Part model, mm, in its own coordinate system. Face numbers are marked on the shaded views. Give positions to 0.01 mm unless a question says otherwise; leave off trailing zeros. Write each loop counter-clockwise with the first axis right and the second up, starting at its lowest first coordinate (ties: lowest second). Pieces come first, ordered by that corner, then holes. Notation, with made-up numbers: M 88.25,-32.5 L 128.25,-32.5 A18 ccw 128.25,-26.5 Z; hole C 13,12 d1. An arc over 180 degrees is marked long. Use a Markdown table: item, result. Add a question column.
from build123d import *

# Parameters (mm, degrees)
F0_R         = 75.9313176518
F0_R_2       = 63.6217413668
F1_DEPTH     = 8.128
F2_DEPTH     = 11.43
F3_R         = 8.1097941577
F4_DEPTH     = 100.33
F5_DEPTH     = 117.094
F6_R         = 8.1153
F7_DEPTH     = 85.852
F8_DEPTH     = 117.094
F9_T2_ANGLE  = 87.3226513318
F9_T4_ANGLE  = 87.3226513318
F9_T6_ANGLE  = 87.3226513318
F9_T8_ANGLE  = 87.3226513318
F10_T2_ANGLE = 92.5127162525
F10_T4_ANGLE = 92.5127162525
F10_T6_ANGLE = 92.5127162525
F10_T8_ANGLE = 92.5127162525


# Not quite as in the source:
# - a fillet or chamfer that OpenCascade refuses, or shapes differently, is made with other operations: its cross-section is extruded or revolved along the edge and cut away or added


with BuildPart() as f1:
    # F0 (on Top) → F1 (new body)
    with BuildSketch(Plane.XY):
        Circle(F0_R)
        Circle(F0_R_2, mode=Mode.SUBTRACT)
        Circle(F0_R_2)
    extrude(amount=-F1_DEPTH)

    # F0 (on Top) → F2 (join)
    with BuildSketch(Plane.XY):
        Circle(F0_R)
        Circle(F0_R_2, mode=Mode.SUBTRACT)
    extrude(amount=F2_DEPTH)

    # F3 (on Right) → F4 (cut)
    with BuildSketch(Plane.YZ):
        with Locations((0, 11.5122310817)):
            Circle(F3_R)
    extrude(amount=-F4_DEPTH, mode=Mode.SUBTRACT)

    # F3 (on Right) → F5 (cut)
    with BuildSketch(Plane.YZ):
        with Locations((0, 11.5122310817)):
            Circle(F3_R)
    extrude(amount=F5_DEPTH, mode=Mode.SUBTRACT)

    # F6 (on Front) → F7 (cut)
    with BuildSketch(Plane.XZ):
        with Locations((0, 11.1844760826)):
            Circle(F6_R)
    extrude(amount=-F7_DEPTH, mode=Mode.SUBTRACT)

    # F6 (on Front) → F8 (cut, symmetric)
    with BuildSketch(Plane.XZ):
        with Locations((0, 11.1844760826)):
            Circle(F6_R)
    extrude(amount=F8_DEPTH, both=True, mode=Mode.SUBTRACT)

    # F9: fillet of radius 2.54 on 4 edges, made by hand

    # F9_s1 → F9_t2 (revolve, cut)
    with BuildSketch(Plane(origin=(0, 0, 0), x_dir=(0, 0, 1), z_dir=(-0.999726726, -0.0233767669, 0))):
        with BuildLine():
            ThreePointArc((8.89, -75.9313176518), (10.6860512242, -75.187368876), (11.43, -73.3913176518))
            Line((11.43, -73.3913176518), (11.43, -75.9313176518))
            Line((11.43, -75.9313176518), (8.89, -75.9313176518))
        make_face()
    revolve(axis=Axis((0, 0, 11.43), (0, 0, 1)), revolution_arc=F9_T2_ANGLE, mode=Mode.SUBTRACT)

    # F9_s3 → F9_t4 (revolve, cut)
    with BuildSketch(Plane(origin=(0, 0, 0), x_dir=(0, 0, 1), z_dir=(-0.0233475312, 0.9997274092, 0))):
        with BuildLine():
            ThreePointArc((8.89, -75.9313176518), (10.6860512242, -75.187368876), (11.43, -73.3913176518))
            Line((11.43, -73.3913176518), (11.43, -75.9313176518))
            Line((11.43, -75.9313176518), (8.89, -75.9313176518))
        make_face()
    revolve(axis=Axis((0, 0, 11.43), (0, 0, 1)), revolution_arc=F9_T4_ANGLE, mode=Mode.SUBTRACT)

    # F9_s5 → F9_t6 (revolve, cut)
    with BuildSketch(Plane(origin=(0, 0, 0), x_dir=(0, 0, 1), z_dir=(0.999726726, 0.0233767669, 0))):
        with BuildLine():
            ThreePointArc((8.89, -75.9313176518), (10.6860512242, -75.187368876), (11.43, -73.3913176518))
            Line((11.43, -73.3913176518), (11.43, -75.9313176518))
            Line((11.43, -75.9313176518), (8.89, -75.9313176518))
        make_face()
    revolve(axis=Axis((0, 0, 11.43), (0, 0, 1)), revolution_arc=F9_T6_ANGLE, mode=Mode.SUBTRACT)

    # F9_s7 → F9_t8 (revolve, cut)
    with BuildSketch(Plane(origin=(0, 0, 0), x_dir=(0, 0, 1), z_dir=(0.0233475312, -0.9997274092, 0))):
        with BuildLine():
            ThreePointArc((8.89, -75.9313176518), (10.6860512242, -75.187368876), (11.43, -73.3913176518))
            Line((11.43, -73.3913176518), (11.43, -75.9313176518))
            Line((11.43, -75.9313176518), (8.89, -75.9313176518))
        make_face()
    revolve(axis=Axis((0, 0, 11.43), (0, 0, 1)), revolution_arc=F9_T8_ANGLE, mode=Mode.SUBTRACT)

    # F10: fillet of radius 3.81 on 4 edges, made by hand

    # F10_s1 → F10_t2 (revolve, cut)
    with BuildSketch(Plane(origin=(0, 0, 0), x_dir=(0, 0, 1), z_dir=(-0.9997599835, 0.0219083392, 0))):
        with BuildLine():
            ThreePointArc((11.43, -67.4317413668), (10.3140768363, -64.7376645305), (7.62, -63.6217413668))
            Line((7.62, -63.6217413668), (11.43, -63.6217413668))
            Line((11.43, -63.6217413668), (11.43, -67.4317413668))
        make_face()
    revolve(axis=Axis((0, 0, 11.43), (0, 0, 1)), revolution_arc=F10_T2_ANGLE, mode=Mode.SUBTRACT)

    # F10_s3 → F10_t4 (revolve, cut)
    with BuildSketch(Plane(origin=(0, 0, 0), x_dir=(0, 0, 1), z_dir=(-0.0219433183, -0.9997592164, 0))):
        with BuildLine():
            ThreePointArc((7.62, -63.6217413668), (10.3140768363, -64.7376645305), (11.43, -67.4317413668))
            Line((11.43, -67.4317413668), (11.43, -63.6217413668))
            Line((11.43, -63.6217413668), (7.62, -63.6217413668))
        make_face()
    revolve(axis=Axis((0, 0, 11.43), (0, 0, 1)), revolution_arc=F10_T4_ANGLE, mode=Mode.SUBTRACT)

    # F10_s5 → F10_t6 (revolve, cut)
    with BuildSketch(Plane(origin=(0, 0, 0), x_dir=(0, 0, 1), z_dir=(0.9997599835, -0.0219083392, 0))):
        with BuildLine():
            ThreePointArc((7.62, -63.6217413668), (10.3140768363, -64.7376645305), (11.43, -67.4317413668))
            Line((11.43, -67.4317413668), (11.43, -63.6217413668))
            Line((11.43, -63.6217413668), (7.62, -63.6217413668))
        make_face()
    revolve(axis=Axis((0, 0, 11.43), (0, 0, 1)), revolution_arc=F10_T6_ANGLE, mode=Mode.SUBTRACT)

    # F10_s7 → F10_t8 (revolve, cut)
    with BuildSketch(Plane(origin=(0, 0, 0), x_dir=(0, 0, 1), z_dir=(0.0219433183, 0.9997592164, 0))):
        with BuildLine():
            ThreePointArc((7.62, -63.6217413668), (10.3140768363, -64.7376645305), (11.43, -67.4317413668))
            Line((11.43, -67.4317413668), (11.43, -63.6217413668))
            Line((11.43, -63.6217413668), (7.62, -63.6217413668))
        make_face()
    revolve(axis=Axis((0, 0, 11.43), (0, 0, 1)), revolution_arc=F10_T8_ANGLE, mode=Mode.SUBTRACT)


solid = f1.part
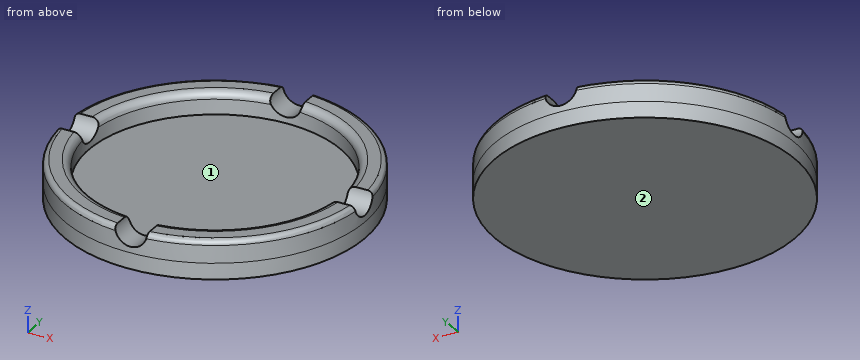
1. Cut at A-A (x = 0). Write the cut outline in (y, z).
2. Drill centre lines: probe 1 along X at (y, z) = (0, 3); probe 2 along Z at (x, y) = (19.5, -14.5). Where is each one in solid material? Low to high. Write a range as [from, to].
3. Flat gauge pins, fed straight in: pin 1 (5 mm diameter, centred on y = 54.5, z = 6.5, fed in from +X); pin 2 (2 mm diameter, centred on x = 16.5, z = 1.5, fed in from -Y); pin 3 (4 mm diameter, centred on y = 42, z = 5, fed in from -X). Where does each tip first touch, or does it go through?
4. Cut at B-B (y = 0). Write the cut outline in (x, z).
5. Cut at C-C (z = -3). Write the cut outline in (x, y), then the cut area to 3 significant figures.
6. Mould opens along Y. For the marked faces 1 and 2 say: released by +Y, released by -Y, zero draft, split by the parting line, or undercut.
A:
| question | item | result |
|---|---|---|
| 1 | outline | M -75.93,-8.13 L 75.93,-8.13 L 75.93,3.07 L 63.62,3.07 L 63.62,0 L -63.62,0 L -63.62,3.07 L -75.93,3.07 Z |
| 2 | probe 1 | x = [-75.93, -63.62], [63.62, 75.93] |
| 2 | probe 2 | z = [-8.13, 0] |
| 3 | pin 1 | stops at x = 55.33 |
| 3 | pin 2 | stops at y = -74.33 |
| 3 | pin 3 | stops at x = -64.54 |
| 4 | outline | M -75.93,-8.13 L 75.93,-8.13 L 75.93,3.4 L 63.62,3.4 L 63.62,0 L -63.62,0 L -63.62,3.4 L -75.93,3.4 Z |
| 5 | outline | C 0,0 d151.86 |
| 5 | area | 18,100 mm² |
| 6 | face 1 | undercut |
| 6 | face 2 | zero draft |
